Input: part model. Units: mm. Frame: model coordinates. Coordinates: 2 decimals unless noted, no trailing zeros. Order: outer loops, then holes, each group sorted by start corner. A loop starts at its lowest first (then second) coordinate and runs counter-clockwise, first axis right, second up. Notation, with made-up numbers: (-16, 82.5) - (9, 82.5) arc R13 ccw to (9, 94.5) - close; hole circle Ø5 at (87.25, -39). An arc over 180 degrees is marked (long way). One line per question, with ' | ' between items.
from build123d import *

# Parameters (mm, degrees)
BOSS_EXTRUDE1_DEPTH = 3.0988
CUT_EXTRUDE1_REACH  = 53.777
SKETCH2_R           = 13.85
CUT_EXTRUDE2_REACH  = 53.777
SKETCH3_W           = 25.4
SKETCH3_H           = 5.715
CUT_EXTRUDE4_REACH  = 53.777
CUT_EXTRUDE5_REACH  = 53.777
SKETCH6_W           = 6.604
SKETCH6_H           = 10.16


with BuildPart() as part:
    # Sketch1 → Boss-Extrude1 (new body)
    with BuildSketch(Plane.XY):
        with BuildLine():
            Line((30.48, -11.260079969), (-30.48, -11.260079969))
            Line((-30.48, -11.260079969), (-30.48, 11.260079969))
            ThreePointArc((-30.48, 11.260079969), (0, 41.740079969), (30.48, 11.260079969))
            Line((30.48, 11.260079969), (30.48, -11.260079969))
        make_face()
    extrude(amount=BOSS_EXTRUDE1_DEPTH)

    # Sketch2 → Cut-Extrude1 (cut, up to next)
    with BuildSketch(Plane.XY.offset(3.0988), mode=Mode.PRIVATE) as cut_extrude1_sk1:
        with Locations((0, 19.504919969)):
            Circle(SKETCH2_R)
    cut_extrude1_tool1 = extrude(cut_extrude1_sk1.sketch, amount=-CUT_EXTRUDE1_REACH, mode=Mode.PRIVATE) & part.part
    add(cut_extrude1_tool1.solids().sort_by_distance((0, 19.50492, 3.0988))[0], mode=Mode.SUBTRACT)

    # Sketch3 → Cut-Extrude2 (cut, up to next)
    with BuildSketch(Plane.XY.offset(3.0988), mode=Mode.PRIVATE) as cut_extrude2_sk1:
        with Locations((0, -8.402579969)):
            Rectangle(SKETCH3_W, SKETCH3_H)
    cut_extrude2_tool1 = extrude(cut_extrude2_sk1.sketch, amount=-CUT_EXTRUDE2_REACH, mode=Mode.PRIVATE) & part.part
    add(cut_extrude2_tool1.solids().sort_by_distance((0, -8.40258, 3.0988))[0], mode=Mode.SUBTRACT)

    # Sketch5 → Cut-Extrude4 (cut, up to next)
    with BuildSketch(Plane.XY.offset(3.0988), mode=Mode.PRIVATE) as cut_extrude4_sk1:
        Polygon((3.175, -1.735079969), (1.143, -1.735079969), (1.143, -5.545079969), (-1.143, -5.545079969), (-1.143, -1.735079969), (-3.175, -1.735079969), (-3.175, 0.804920031), (-1.143, 0.804920031), (-1.143, 8.424920031), (1.143, 8.424920031), (1.143, 0.804920031), (3.175, 0.804920031), align=None)
    cut_extrude4_tool1 = extrude(cut_extrude4_sk1.sketch, amount=-CUT_EXTRUDE4_REACH, mode=Mode.PRIVATE) & part.part
    add(cut_extrude4_tool1.solids().sort_by_distance((0, 0.974577, 3.0988))[0], mode=Mode.SUBTRACT)

    # Sketch6 → Cut-Extrude5 (cut, up to next)
    with BuildSketch(Plane.XY.offset(3.0988), mode=Mode.PRIVATE) as cut_extrude5_sk1:
        with Locations((22.86, 7.710464847)):
            Rectangle(SKETCH6_W, SKETCH6_H)
    cut_extrude5_tool1 = extrude(cut_extrude5_sk1.sketch, amount=-CUT_EXTRUDE5_REACH, mode=Mode.PRIVATE) & part.part
    # Sketch6 → Cut-Extrude5 (cut, up to next)
    with BuildSketch(Plane.XY.offset(3.0988), mode=Mode.PRIVATE) as cut_extrude5_sk2:
        with Locations((-22.86, 7.710464847)):
            Rectangle(SKETCH6_W, SKETCH6_H)
    cut_extrude5_tool2 = extrude(cut_extrude5_sk2.sketch, amount=-CUT_EXTRUDE5_REACH, mode=Mode.PRIVATE) & part.part
    add(cut_extrude5_tool1.solids().sort_by_distance((22.86, 7.710465, 3.0988))[0], mode=Mode.SUBTRACT)
    add(cut_extrude5_tool2.solids().sort_by_distance((-22.86, 7.710465, 3.0988))[0], mode=Mode.SUBTRACT)


solid = part.part
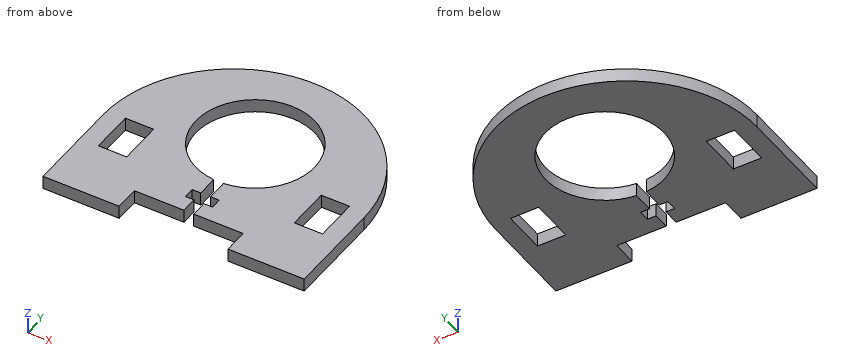
Item 1: Section A-A on y = -0.5. Return the cut outline in (x, z) (3 decimals).
Data:
outline: (-30.48, 0) - (-3.175, 0) - (-3.175, 3.099) - (-30.48, 3.099) - close; (3.175, 0) - (30.48, 0) - (30.48, 3.099) - (3.175, 3.099) - close
Item 2: Ray query, line 1 (X direction, y = 4, z = 2.5); line 2 (X direction, y = -3.5, z = 0.45); line 3 (X direction, y = 31, z = 1.6). Return the intervals inside material, ascending.
Data:
line 1: -30.48 to -26.16, -19.56 to -1.14, 1.14 to 19.56, 26.16 to 30.48 | line 2: -30.48 to -1.14, 1.14 to 30.48 | line 3: -23.22 to -7.73, 7.73 to 23.22
Item 3: Section C-C on x = -11.5. Return the cut outline in (y, z).
Data:
outline: (-5.55, 0) - (11.79, 0) - (11.79, 3.1) - (-5.55, 3.1) - close; (27.22, 0) - (39.49, 0) - (39.49, 3.1) - (27.22, 3.1) - close
Item 4: Section B-B on z = 1.25. Return the cut outline in (x, y) (3 decimals).
Data:
outline: (-30.48, -11.26) - (-12.7, -11.26) - (-12.7, -5.545) - (-1.143, -5.545) - (-1.143, -1.735) - (-3.175, -1.735) - (-3.175, 0.805) - (-1.143, 0.805) - (-1.143, 5.702) arc R13.85 cw (long way) to (1.143, 5.702) - (1.143, 0.805) - (3.175, 0.805) - (3.175, -1.735) - (1.143, -1.735) - (1.143, -5.545) - (12.7, -5.545) - (12.7, -11.26) - (30.48, -11.26) - (30.48, 11.26) arc R30.48 ccw to (-30.48, 11.26) - close; hole (-26.162, 2.63) - (-19.558, 2.63) - (-19.558, 12.79) - (-26.162, 12.79) - close; hole (19.558, 2.63) - (26.162, 2.63) - (26.162, 12.79) - (19.558, 12.79) - close
Item 5: Contact query for flat-ended pins moving along their axis: P1, Ø1.6, axis at x = -2.5, z = 1, coming from the -Y side; P2, Ø0.9, axis at x = -23, z = 2, coming from the +Y side; P3, Ø1, axis at y = 19, z = 1.5, coming from the -X side; P4, Ø25, axis at x = 0, y = 19.5, coming from the +Z side. Output: stop coordinate, or through.
Data:
P1: y = -5.55 | P2: y = 31.77 | P3: x = -29.61 | P4: through
Item 6: Section D-D on x = 0. Return the cut outline in (y, z).
Data:
outline: (33.35, 0) - (41.74, 0) - (41.74, 3.1) - (33.35, 3.1) - close
